Input: part model. Units: mm. Frame: model coordinates. Coordinates: 2 decimals unless noted, no trailing zeros. Loops run counter-clockwise (first coordinate to the right, second up) from the corner with the lowest first, then second, coordinate; pieces in that order, holes last.
(1) Mould query, pull axis X, two halves, no side actions, for faces 1 (the face through (1.8, 8.6, 27.9)), 2 (the face through (-0.414, 3.154, 5.07)), 3 (the face through (0, 8, 20)). Classes: released by +X, released by -X, zero draft, split by the parting line, or undercut.
(2) Section C-C, the plane z = 29. Return loops of the section in (x, y).
(3) Contact query for flat-ended pins moving along their axis: P1, Ø1.5, axis at x = -3.5, z = 33, coming from the +Y side; P2, Ø5.5, axis at y = 9, z = 26, coming from the -X side. Output: stop coordinate, or through.
(4) Section A-A, the plane y = 0. Return loops of the section in (x, z), then the cut area to 3 significant figures.
(5) Section B-B, the plane z = 16. Return loops of the section in (x, y), then the cut area to 3 significant figures.
(6) Line query: L1, parallel to X at y = 0, z = 23.25; L2, parallel to Y at x = -2, z = 21; L3, parallel to X at y = 8.25, z = 15. Output: solid intervals per line, ascending.
(7) Section D-D, the plane y = 8. Return loops of the section in (x, z).
```python
from build123d import *

# Parameters (mm, degrees)
BOSS_EXTRUDE1_DEPTH = 40
SKETCH2_R           = 2.1
CUT_EXTRUDE1_DEPTH  = 42.990351999
CHAMFER1_SIZE       = 10
CHAMFER1_SIZE2      = 0.874886635


with BuildPart() as part:
    # Sketch1 → Boss-Extrude1 (new body)
    with BuildSketch(Plane.XY):
        Polygon((-4.25, -4), (-4.25, 3.5), (0, 5.046873496), (0, 12.046873496), (3.75, 12.046873496), (3.75, -4), align=None)
        with BuildLine():
            ThreePointArc((2.75, 0), (0, 2.75), (-2.75, 0))
            ThreePointArc((-2.75, 0), (0, -2.75), (2.75, 0))
        make_face(mode=Mode.SUBTRACT)
    extrude(amount=BOSS_EXTRUDE1_DEPTH)

    # Sketch2 → Cut-Extrude1 (cut, through all)
    with BuildSketch(Plane.ZY):
        with Locations((10, 8.546873496)):
            Circle(SKETCH2_R)
        with Locations((30, 8.546873496)):
            Circle(SKETCH2_R)
    extrude(amount=-CUT_EXTRUDE1_DEPTH, mode=Mode.SUBTRACT)

    # Chamfer1
    chamfer1_edges = [part.edges().sort_by_distance(p)[0] for p in [
        (-2.75, 0, 40),
    ]]
    chamfer1_side = [part.faces().sort_by_distance(p)[0] for p in [
        (-2.75, 0, 20),
    ]]
    chamfer(chamfer1_edges, length=CHAMFER1_SIZE, length2=CHAMFER1_SIZE2, reference=chamfer1_side[0])

    # Chamfer2: read off the stored shape, not the designer's step
    # Chamfer2 outline → Chamfer2 (revolve, cut)
    with BuildSketch(Plane.XZ):
        Polygon((3.624886635, 0), (2.75, 10), (2.75, 0), align=None)
    revolve(axis=Axis((0, 0, 0), (0, 0, 1)), mode=Mode.SUBTRACT)


solid = part.part
```
Report:
1. face 1: zero draft
1. face 2: undercut
1. face 3: released by -X
2. outline: (-4.25, -4) - (3.75, -4) - (3.75, 6.7) - (0, 6.7) - (0, 5.05) - (-4.25, 3.5) - close; (0, 10.39) - (3.75, 10.39) - (3.75, 12.05) - (0, 12.05) - close; hole circle Ø5.5 at (0, 0)
3. P1: stops at y = 4.05
3. P2: stops at x = 0
4. outline: (-4.25, 0) - (-3.62, 0) - (-2.75, 10) - (-2.75, 30) - (-3.62, 40) - (-4.25, 40) - close; (2.75, 10) - (3.62, 0) - (3.75, 0) - (3.75, 40) - (3.62, 40) - (2.75, 30) - close
4. area: 82.5 mm2
5. outline: (-4.25, -4) - (3.75, -4) - (3.75, 12.05) - (0, 12.05) - (0, 5.05) - (-4.25, 3.5) - close; hole circle Ø5.5 at (0, 0)
5. area: 71.6 mm2
6. L1: x = -4.25 to -2.75, 2.75 to 3.75
6. L2: y = -4 to -1.89, 1.89 to 4.32
6. L3: x = 0 to 3.75
7. outline: (0, 0) - (3.75, 0) - (3.75, 7.97) - (0, 7.97) - close; (0, 12.03) - (3.75, 12.03) - (3.75, 27.97) - (0, 27.97) - close; (0, 32.03) - (3.75, 32.03) - (3.75, 40) - (0, 40) - close
